For this review, use the dimensioned drawing (mm, ordinates from the lowest corner) and the shaded views. A direction names the side the tool comes from. Give positions to 0.01 mm unless a question says otherwise; leave off trailing zeros. Order: outer loops, then holes, each group sorted by start corner. A loop starts at its lowest first (then second) coordinate and runs counter-clockwise, first axis right, second up. Notation, with made-up numbers: (-6.75, 20.5) - (0.25, 20.5) arc R5 cw to (0.25, 24.5) - close; hole circle Ø10 at (-27, 50). An arc over 180 degrees is marked (long way). One line per item, written item: value.
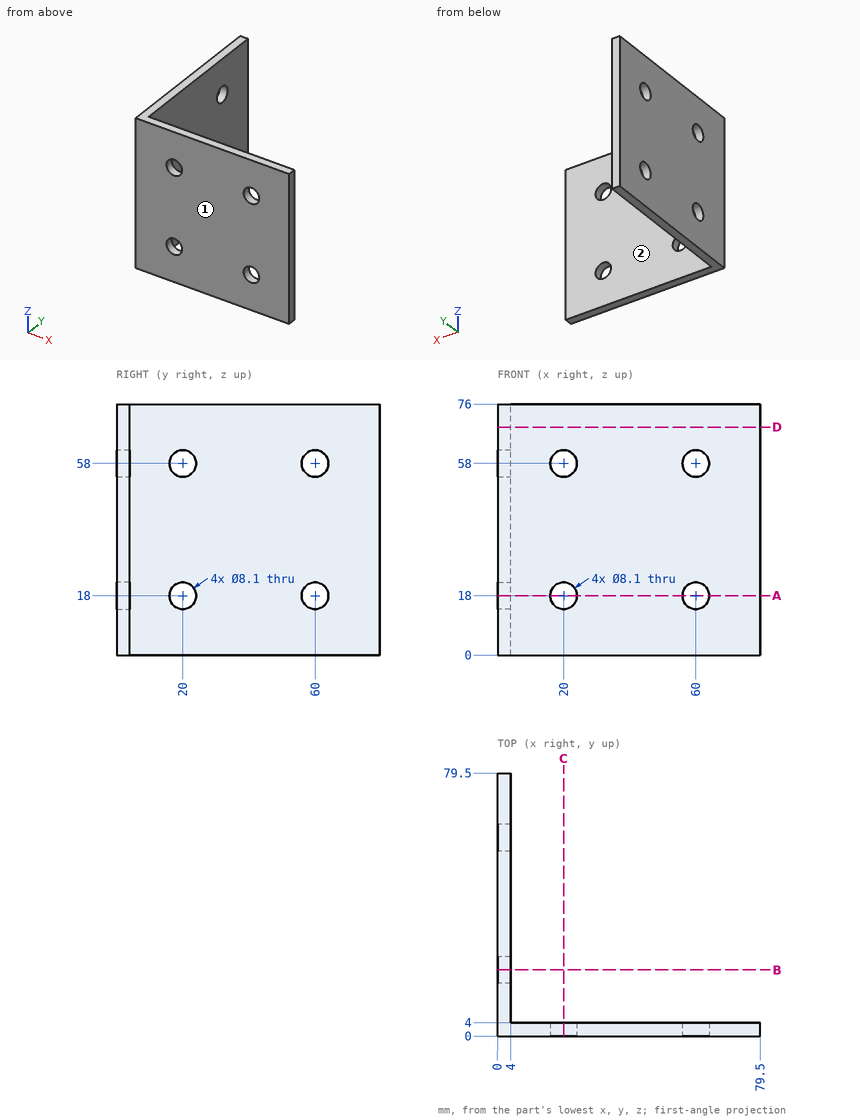
(1) Take a section at D-D (z = 69). Write out the cut boundary in (x, y), then the cut area to 3 significant figures.
Answers below:
outline: (0, 0) - (79.5, 0) - (79.5, 4) - (4, 4) - (4, 79.5) - (0, 79.5) - close
area: 620 mm^2
(2) Take a section at A-A (z = 18). Write out the cut boundary in (x, y), then the cut area to 3 significant figures.
Answers below:
outline: (0, 0) - (15.95, 0) - (15.95, 4) - (4, 4) - (4, 15.95) - (0, 15.95) - close; (0, 24.05) - (4, 24.05) - (4, 55.95) - (0, 55.95) - close; (0, 64.05) - (4, 64.05) - (4, 79.5) - (0, 79.5) - close; (24.05, 0) - (55.95, 0) - (55.95, 4) - (24.05, 4) - close; (64.05, 0) - (79.5, 0) - (79.5, 4) - (64.05, 4) - close
area: 490 mm^2
(3) Wall thickness on line 1 (Y direction, x = 2, z = 18); line 2 (Z direction, x = 3, y = 20): over which ranges is each line inside the solid? List them lowest first. Write a range as from..to.
Answers below:
line 1: y = 0..15.95, 24.05..55.95, 64.05..79.5
line 2: z = 0..13.95, 22.05..53.95, 62.05..76
(4) Machinability: for the marked faces 1 and 2, which of the approach directions +Z, -Z, +X, -X, +Y, -Y give a long, thin tool a straight path to every point of the face, cutting with its end or side? Answer none if there is none.
Answers below:
face 1: +Z, -Z, +X, -X, -Y
face 2: +Z, -Z, +X, +Y
(5) Take a section at B-B (y = 20). Write out the cut boundary in (x, z), then the cut area to 3 significant figures.
Answers below:
outline: (0, 0) - (4, 0) - (4, 13.95) - (0, 13.95) - close; (0, 22.05) - (4, 22.05) - (4, 53.95) - (0, 53.95) - close; (0, 62.05) - (4, 62.05) - (4, 76) - (0, 76) - close
area: 239 mm^2
(6) For P1, Ø5, axis at y = 53.5, z = 36, coming from the +X side; P2, Ø9.5, axis at x = 20, z = 18, coming from the +Y side, all flat-tipped, find the tip position at first contact; note any pin that passes through.
Answers below:
P1: stops at x = 4
P2: stops at y = 4
